Read the model definition and answer for the solid it produces. Units are mm, in the model's axes. A direction names the side the tool comes from. Give positions to 0.01 mm unless a question says otherwise; leave off trailing zeros. Order: outer loops, then holes, each group sorted by start corner. A loop starts at its lowest first (then second) coordinate and runs counter-clockwise, first axis right, second up.
```python
from build123d import *

# Parameters (mm, degrees)
F0_W     = 15
F0_H     = 10
F0_R     = 3.5
F1_DEPTH = 5
F0_W_2   = 3
F2_DEPTH = 2
F3_R     = 0.99999
F0_R_2   = 2
F4_DEPTH = 5
F5_SIZE  = 1.5


# Not quite as in the source:
# - a fillet or chamfer is up to 0.001 mm smaller than in the source, because OpenCascade refuses the exact size


with BuildPart() as f1:
    # F0 (on Top) → F1 (new body)
    with BuildSketch(Plane.XY):
        with Locations((7.5, -5)):
            Rectangle(F0_W, F0_H)
        with Locations((7.5, -5)):
            Circle(F0_R, mode=Mode.SUBTRACT)
    extrude(amount=F1_DEPTH)

    # F0 (on Top) → F2 (join)
    with BuildSketch(Plane.XY):
        with Locations((-1.5, -5)):
            Rectangle(F0_W_2, F0_H)
        with Locations((16.5, -5)):
            Rectangle(F0_W_2, F0_H)
    extrude(amount=F2_DEPTH)

    # F3 (radius 1 in the source; OpenCascade refuses exactly that, so slightly less here)
    f3_edges = [f1.edges().sort_by_distance(p)[0] for p in [
        (15, 0, 3.5),
        (7.5, 0, 5),
        (0, 0, 3.5),
        (-1.5, 0, 2),
        (-3, 0, 1),
        (7.5, 0, 0),
        (18, 0, 1),
        (16.5, 0, 2),
        (0, -10, 3.5),
        (7.5, -10, 5),
        (15, -10, 3.5),
        (16.5, -10, 2),
        (18, -10, 1),
        (7.5, -10, 0),
        (-3, -10, 1),
        (-1.5, -10, 2),
        (15, -5, 2),
        (15, -5, 5),
        (18, -5, 0),
        (18, -5, 2),
        (0, -5, 2),
        (-3, -5, 2),
        (0, -5, 5),
        (-3, -5, 0),
    ]]
    fillet(f3_edges, radius=F3_R)

    # F0 (on Top) → F4 (join)
    with BuildSketch(Plane.XY):
        with Locations((7.5, -5)):
            Circle(F0_R)
        with Locations((7.5, -5)):
            Circle(F0_R_2, mode=Mode.SUBTRACT)
    extrude(amount=F4_DEPTH)

    # F5
    f5_edges = [f1.edges().sort_by_distance(p)[0] for p in [
        (5.5, -5, 0),
    ]]
    chamfer(f5_edges, length=F5_SIZE)


solid = f1.part
```
1) A tool of negligible diameter and unlimited length cuts with its end or side. For faces 5 (the face through (7, -10, 2)), 6 (the face through (16.507, -0.301, 1.715)), 7 (the face through (-1.5, -4.9, 2)), 8 (the face through (-1.493, -9.699, 1.715)), 9 (the face through (-1.493, -0.301, 1.715)), from which of +Z, -Z, +X, -X, +Y, -Y can it reach the whole face along a straight path? Write none if from no direction.
Final values:
face 5: +Z, -Z, +X, -X, -Y
face 6: +Z, +X, +Y
face 7: +Z, -X, +Y, -Y
face 8: +Z, -X, -Y
face 9: +Z, -X, +Y
2) The part is cut by section C-C on z = 3.2. Determine the outline of the cut face in (x, y), and give its area (3 significant figures).
Final values:
outline: (0, -9) arc R1 ccw to (1, -10) - (14, -10) arc R1 ccw to (15, -9) - (15, -1) arc R1 ccw to (14, 0) - (1, 0) arc R1 ccw to (0, -1) - close; hole circle Ø4 at (7.5, -5)
area: 137 mm2
3) Given pin 1 (0.5 mm diameter, centred on x = -1.5, y = -3.5, fed in from +Z); pin 2 (2 mm diameter, centred on y = -6.5, z = 4, fed in from +X); pin 3 (0.5 mm diameter, centred on y = -4, z = 3.5, fed in from -X), each flat-ended and moving along its own axis, determine where each tip first touches the part or whether it passes through.
Final values:
pin 1: stops at z = 2
pin 2: stops at x = 15
pin 3: stops at x = 0
4) The part is cut by section D-D on x = 2.5. Determine the outline of the cut face in (y, z).
Final values:
outline: (-10, 1) arc R1 ccw to (-9, 0) - (-1, 0) arc R1 ccw to (0, 1) - (0, 4) arc R1 ccw to (-1, 5) - (-9, 5) arc R1 ccw to (-10, 4) - close
5) The part is cut by section B-B on x = 7.5. Determine the outline of the cut face in (y, z), and give its area (3 significant figures).
Final values:
outline: (-10, 1) arc R1 ccw to (-9, 0) - (-8.5, 0) - (-7, 1.5) - (-7, 5) - (-9, 5) arc R1 ccw to (-10, 4) - close; (-3, 1.5) - (-1.5, 0) - (-1, 0) arc R1 ccw to (0, 1) - (0, 4) arc R1 ccw to (-1, 5) - (-3, 5) - close
area: 26.9 mm2
6) Consider L1, parallel to Y at x = 7.5, z = 3.9; L2, parallel to X at y = -4.75, z = 1.4; L3, parallel to X at y = -6.5, z = 2.7. Determine where each line is inside the solid, lowest interval first.
Final values:
L1: y = -10 to -7, -3 to 0
L2: x = -2.92 to 5.41, 9.59 to 17.92
L3: x = -0.05 to 6.18, 8.82 to 15.05
7) For a pull along X with two mould halves and no side action, classify faces 1 (the face through (6, -3, 5)), 2 (the face through (5.9, -6.2, 3.2)), 3 (the face through (15, -5.1, 3.5)), 4 (the face through (-2.715, -4.944, 1.699)) as released by +X, released by -X, zero draft, split by the parting line, or undercut.
Final values:
face 1: zero draft
face 2: undercut
face 3: released by +X
face 4: released by -X
